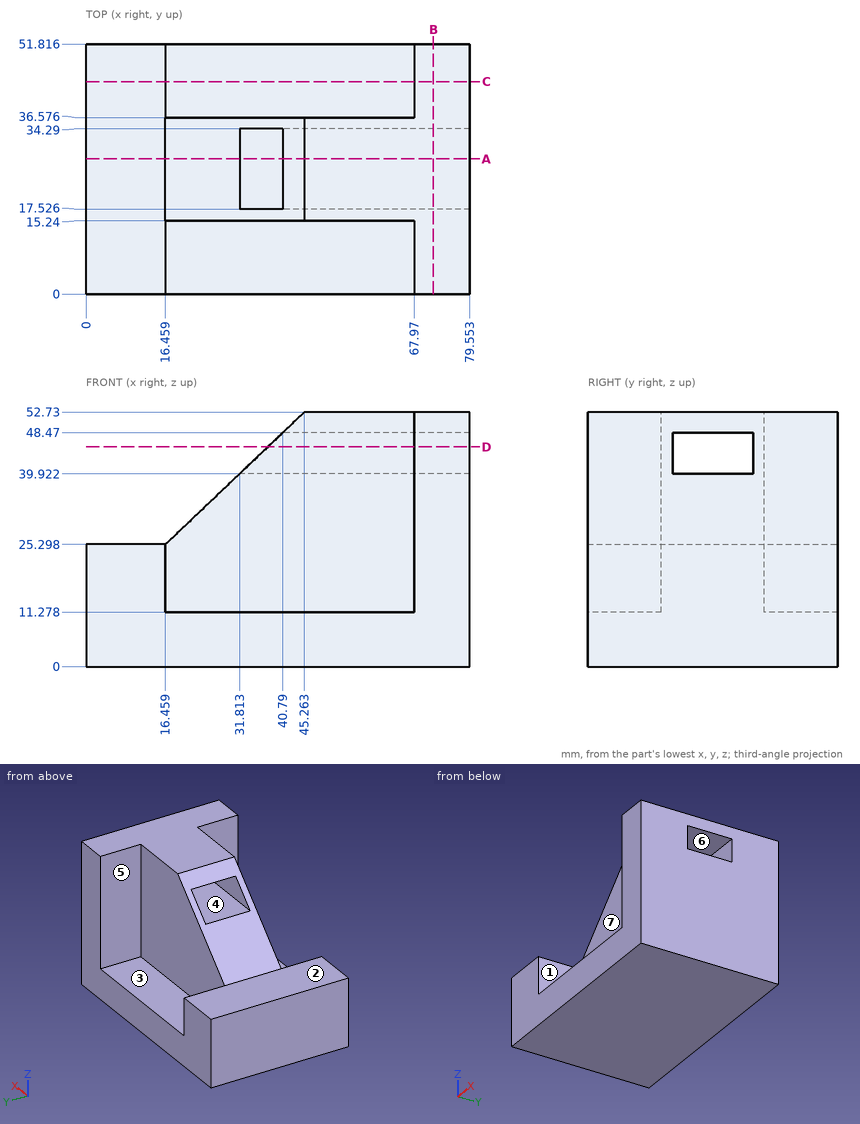
Study the drawing (mm; zero at the part's minimum x, y, z) and answer. A direction names the side the tool comes from. Coordinates: 2 decimals unless noted, no trailing zeros. Loops run counter-clockwise (first coordinate to the right, second up) from the corner with the lowest first, then second, coordinate; pieces in that order, holes last. Notation, with made-up numbers: M 8.5,1.5 L 30.5,1.5 A17 cw 30.5,15.5 Z; hole C 66,-25 d1. An arc over 180 degrees is marked long. Answer as a JSON object with one key per item and string values. Group by question number.
Item 1: Section C-C (y = 44) is taken. Write down the section's boundary in (x, z), and give its area (3 significant figures).
Item 2: Each of these flat-tipped pins is pushed along its axis until it touches: P1, Ø17, axis at x = 47, y = 9, coming from the +Z side; P2, Ø4, axis at x = 18, y = 6, coming from the +Z side; P3, Ø12.5, axis at x = 50, z = 38, coming from the +Y side; P4, Ø1, axis at x = 33, z = 30, coming from the -Y side. Where does it stop, or does it pass through?
Item 3: Section B-B (x = 72) is taken. Write down the section's boundary in (y, z).
Item 4: Determine the mould class of the marked faces 5, 6 and 7 for opening direction Y: +Y half, -Y half, draft (parallel to the pull), parting line (faces both ways), or undercut.
Item 5: Section D-D (z = 45.5) is taken. Write down the section's boundary in (x, y).
Item 6: Consider L1, parallel to X at y = 45.5, z = 12; L2, parallel to Z at x = 67, y = 28; L3, parallel to Y at x = 48, z = 44. Determine where each line is inside the solid, lowest interval first.
Item 7: Which of the six approach directions +Z, -Z, +X, -X, +Y, -Y give full straight-line access (tool end or side, diameter ignored) to the marked faces 1, 2, 3 and 4?
Item 8: Section A-A (y = 28) is taken. Write down the section's boundary in (x, z).
Solved:
{
 "1": {"outline": "M 0,0 L 79.55,0 L 79.55,52.73 L 67.97,52.73 L 67.97,11.28 L 16.46,11.28 L 16.46,25.3 L 0,25.3 Z", "area": "1,610 mm2"},
 "2": {"P1": "stops at z = 52.73", "P2": "stops at z = 25.3", "P3": "stops at y = 36.58", "P4": "stops at y = 15.24"},
 "3": {"outline": "M 0,0 L 51.82,0 L 51.82,52.73 L 0,52.73 Z; hole M 17.53,39.92 L 34.29,39.92 L 34.29,48.47 L 17.53,48.47 Z"},
 "4": {"face 5": "draft", "face 6": "undercut", "face 7": "-Y half"},
 "5": {"outline": "M 37.67,15.24 L 67.97,15.24 L 67.97,0 L 79.55,0 L 79.55,17.53 L 37.67,17.53 Z; M 37.67,34.29 L 79.55,34.29 L 79.55,51.82 L 67.97,51.82 L 67.97,36.58 L 37.67,36.58 Z"},
 "6": {"L1": "x = 0 to 16.46, 67.97 to 79.55", "L2": "z = 0 to 39.92, 48.47 to 52.73", "L3": "y = 15.24 to 17.53, 34.29 to 36.58"},
 "7": {"face 1": "+Z, -Y", "face 2": "+Z, -X, +Y, -Y", "face 3": "+Z, +Y", "face 4": "+X, -X"},
 "8": {"outline": "M 0,0 L 79.55,0 L 79.55,39.92 L 31.81,39.92 L 16.46,25.3 L 0,25.3 Z; M 40.79,48.47 L 79.55,48.47 L 79.55,52.73 L 45.26,52.73 Z"}
}
